```python
from build123d import *

# Parameters (mm, degrees)
SKETCH1_W           = 70
SKETCH1_H           = 25
BOSS_EXTRUDE1_DEPTH = 45
CUT_EXTRUDE1_DEPTH  = 15
CUT_EXTRUDE2_DEPTH  = 26
SKETCH4_W           = 20
SKETCH4_H           = 10
CUT_EXTRUDE3_DEPTH  = 46
SKETCH5_R           = 5
CUT_EXTRUDE4_DEPTH  = 26


with BuildPart() as part:
    # Sketch1 → Boss-Extrude1 (new body)
    with BuildSketch(Plane(origin=(0, 0, 0), x_dir=(1, 0, 0), z_dir=(0, 1, 0))):
        with Locations((35, 12.5)):
            Rectangle(SKETCH1_W, SKETCH1_H)
    extrude(amount=BOSS_EXTRUDE1_DEPTH)

    # Sketch2 → Cut-Extrude1 (cut)
    with BuildSketch(Plane.XY):
        Polygon((0, 39.67789539), (0, 24.67789539), (70, 10), (70, 25), align=None)
    extrude(amount=-CUT_EXTRUDE1_DEPTH, mode=Mode.SUBTRACT)

    # Sketch3 → Cut-Extrude2 (cut, through all)
    with BuildSketch(Plane.XY):
        Polygon((30, 45), (30, 33.387368794), (70, 25), (70, 45), align=None)
    extrude(amount=-CUT_EXTRUDE2_DEPTH, mode=Mode.SUBTRACT)

    # Sketch4 → Cut-Extrude3 (cut, through all)
    with BuildSketch(Plane(origin=(0, 0, 0), x_dir=(-1, 0, 0), z_dir=(0, -1, 0))):
        with Locations((-45, 5)):
            Rectangle(SKETCH4_W, SKETCH4_H)
    extrude(amount=-CUT_EXTRUDE3_DEPTH, mode=Mode.SUBTRACT)

    # Sketch5 → Cut-Extrude4 (cut, through all)
    with BuildSketch(Plane.XY):
        with Locations((15, 10)):
            Circle(SKETCH5_R)
    extrude(amount=-CUT_EXTRUDE4_DEPTH, mode=Mode.SUBTRACT)


solid = part.part
```
The model under review builds one solid part; all positions refer to its coordinate system, in mm. A direction names the side the tool comes from. Round coordinates to 2 decimals unless told otherwise and drop trailing zeros. Order: outer loops, then holes, each group sorted by start corner. A loop starts at its lowest first (then second) coordinate and runs counter-clockwise, first axis right, second up.
(1) For P1, Ø19, axis at x = 48.5, y = 12.5, coming from the +Z side; P2, Ø3.5, axis at y = 38, z = -16, coming from the +X side; P3, Ø3, axis at x = 38.5, z = -7, coming from the +Y side, all flat-tipped, find the tip position at first contact; note any pin that passes through.
Working result:
P1: stops at z = 0
P2: stops at x = 30
P3: passes through
(2) Tool access review of faces 4 (the face through (35, 9, -5)), 5 (the face through (30, 39, -12)), 6 (the face through (19.77, 11.5, -12.32)), 7 (the face through (15.21, 36.49, -7.4)), 8 (the face through (34.51, 17.44, -7.4)): name each direction out of +Z, -Z, +X, -X, +Y, -Y from which nothing blocks a thin tool from reaching the whole face with its end or side.
Working result:
face 4: +Z, +Y, -Y
face 5: +Z, -Z, +X, +Y
face 6: +Z, -Z
face 7: +Z, -X
face 8: +Z, +X
(3) Take a section at B-B, the plane z = -21.5. State the section outline as (x, y) points, plus the area to 3 significant figures.
Working result:
outline: (0, 0) - (70, 0) - (70, 25) - (30, 33.39) - (30, 45) - (0, 45) - close; hole circle Ø10 at (15, 10)
area: 2,440 mm2
(4) Mouldability with a two-part tool opening along Y and no side actions: class faces 1 (the face through (35, 25, -15)), 2 (the face through (15, 45, -13)), 3 (the face through (70, 9.5, -15.1)) as released by +Y, released by -Y, zero draft, split by the parting line, or undercut.
Working result:
face 1: undercut
face 2: released by +Y
face 3: zero draft
(5) Take a section at D-D, the plane y = 31.5. State the section outline as (x, z) points, plus the area to 3 significant figures.
Working result:
outline: (0, -25) - (39, -25) - (39, -15) - (0, -15) - close
area: 390 mm2
(6) Take a section at A-A, the plane x = 15. State the section outline as (y, z) points, plus the area to 3 significant figures.
Working result:
outline: (0, -25) - (5, -25) - (5, 0) - (0, 0) - close; (15, -25) - (45, -25) - (45, 0) - (36.53, 0) - (36.53, -15) - (21.53, -15) - (21.53, 0) - (15, 0) - close
area: 650 mm2
(7) Take a section at C-C, the plane x = 8. State the section outline as (y, z) points.
Working result:
outline: (0, -25) - (45, -25) - (45, 0) - (38, 0) - (38, -15) - (23, -15) - (23, 0) - (0, 0) - close
(8) Wall thickness on L1, parallel to X at y = 9.5, z = -3; L2, parallel to Y at x = 15, z = -19.5; L3, parallel to Y at x = 15, z = -12.25: over which ranges is each line inside the solid? List them lowest first.
Working result:
L1: x = 0 to 10.03, 19.97 to 35, 55 to 70
L2: y = 0 to 5, 15 to 45
L3: y = 0 to 5, 15 to 21.53, 36.53 to 45
